Autodesk Inventor part; units mm, degrees
ref_plane "YZ Plane" through (0, 0, 0) normal (1, 0, 0) x (0, 1, 0)
ref_plane "XZ Plane" through (0, 0, 0) normal (0, 1, 0) x (-1, 0, 0)
ref_plane "XY Plane" through (0, 0, 0) normal (0, 0, 1) x (1, 0, 0)
sketch "Sketch1" plane through (0, 0, 0) normal (0, 1, 0) x (-1, 0, 0)
  line L0 (0, 4) -> (-20, 4)
  line L1 (-20, 4) -> (-20, -4)
  line L2 (-20, -4) -> (0, -4)
  circle A0 centre (-20, 0) radius 4
  circle A1 centre (-20, 0) radius 2.5
  line L3 (-20, -4) -> (-30, -4)
  line L4 (-30, -4) -> (-30, 4)
  line L5 (-30, 4) -> (-20, 4)
  line L6 (-20, 4) -> (-20, -4)
  circle A2 centre (4, 0) radius 4
  circle A3 centre (4, 0) radius 2.5
  line L7 (0, 4) -> (4, 4)
  line L8 (4, -4) -> (0, -4)
  line L9 (0, 0) -> (-1.5, 0)
  line L10 (-1.5, 0) -> (-14.5, 0)
  line L11 (-14.5, 0) -> (-14.5, -4)
  line L12 (-1.5, 0) -> (-1.5, -4)
  line L13 (-1.5, 0) -> (-1.5, 4)
  line L14 (-14.5, 0) -> (-14.5, 4)
  dimension "d0" = 20
  dimension "d1" = 5
  dimension "d2" = 10
  dimension "d3" = 5
  dimension "d4" = 1.5
  dimension "d5" = 13
extrude "Extrusion1" add sketch "Sketch1" along normal blind 5 contours L13 L10 L14 L0 | L12 L2 L11 L10
sketch "Sketch2" plane through (0, 5, 0) normal (0, 1, 0) x (1, 0, 0)
  line L0 (14.5, 4) -> (1.5, 4)
  line L1 (1.5, 4) -> (1.5, 3)
  line L2 (1.5, 4) -> (1.5, -4)
  line L3 (1.5, 3) -> (1.5, -3)
  line L4 (1.5, 3) -> (14.5, 3)
  line L5 (14.5, 3) -> (14.5, -3)
  line L6 (14.5, -4) -> (14.5, 4)
  line L7 (1.5, -3) -> (14.5, -3)
  line L8 (1.5, -4) -> (14.5, -4)
  line L9 (14.5, -4) -> (1.5, -4)
  point P0 (0, 0)
  dimension "d8" = 1
  dimension "d9" = 6
extrude "Extrusion2" cut sketch "Sketch2" against normal blind 1 contours L6 L4 L1 L0 | L6 L8 L2 L7
properties part number "sensorMount"
Design review of the part built by this model. Coordinates are the model's own, in mm. A direction names the side the tool comes from. Coordinates: 2 decimals unless noted, no trailing zeros. Order: outer loops, then holes, each group sorted by start corner. A loop starts at its lowest first (then second) coordinate and runs counter-clockwise, first axis right, second up. Notation, with made-up numbers: M 12.25,81 L 63.25,81 A32 cw 63.25,116 Z; hole C 25.5,-5 d1. An arc over 180 degrees is marked long. Use a Markdown table: item, result.
(1) Wall thickness on probe 1 along Z at (x, y) = (3, 4.6); probe 2 along Y at (x, z) = (10.5, 3.5): over which ranges is each line inside the solid? List them lowest first.
Worked answers:
| item | result |
|---|---|
| probe 1 | z = -3 to 3 |
| probe 2 | y = 0 to 4 |
(2) For P1, Ø0.8, axis at x = 5.5, z = 3.5, coming from the +Y side; P2, Ø0.8, axis at x = 5.5, y = 4.5, coming from the -Z side, all flat-tipped, find the tip position at first contact; note any pin that passes through.
Worked answers:
| item | result |
|---|---|
| P1 | stops at y = 4 |
| P2 | stops at z = -3 |
(3) Add section B-B (z = 3.5). Give the boundary of the cut face in (x, y), then the cut area to 3 significant figures.
Worked answers:
| item | result |
|---|---|
| outline | M 1.5,0 L 14.5,0 L 14.5,4 L 1.5,4 Z |
| area | 52.0 mm2 |
(4) For faces 1 (the flat face through (7.9, 4.5, -3)), 2 (the flat face through (14.5, 2, 0)), 3 (the flat face through (7.9, 4.5, 3)), list the 3-axis set-ups (+Z, -Z, +X, -X, +Y, -Y) from which the entire face can be reached by the end or side of a thin tool; tool diameter is ignored.
Worked answers:
| item | result |
|---|---|
| face 1 | -Z, +X, -X, +Y |
| face 2 | +Z, -Z, +X, +Y, -Y |
| face 3 | +Z, +X, -X, +Y |
(5) Add section A-A (x = 10.25). Give the boundary of the cut face in (y, z).
Worked answers:
| item | result |
|---|---|
| outline | M 0,-4 L 4,-4 L 4,-3 L 5,-3 L 5,3 L 4,3 L 4,4 L 0,4 Z |
